The model under review builds one solid part; all positions refer to its coordinate system, in mm. Face numbers are marked on the shaded views. A direction names the side the tool comes from. Round coordinates to 2 decimals unless told otherwise and drop trailing zeros. Write each loop counter-clockwise with the first axis right and the second up, starting at its lowest first coordinate (ties: lowest second). Pieces come first, ordered by that corner, then holes. Notation, with made-up numbers: (17.25, 14) -> (53.25, 14) arc R23 ccw to (53.25, 31) -> close; hole circle Ø11 at (-9.5, 32.25). An arc over 180 degrees is marked (long way). Answer as a JSON object with one key per item and string values. Group by question number.
1) Machinability: for the marked faces 1, 2, 3 and 4, which of the approach directions +Z, -Z, +X, -X, +Y, -Y give a long, thin tool a straight path to every point of the face, cutting with its end or side? Answer none if there is none.
2) Mouldability with a two-part tool opening along X and no side actions: class the marked faces 5, 6 and 7 as pulls with the +X half, pulls with the -X half, needs draft (parallel to the pull), parting line crosses it, or undercut.
3) We need section D-D, the plane y = -4.25. Write out the cut boundary in (x, z), then the cut area to 3 significant figures.
4) We need section C-C, the plane z = 0.5. Write out the cut boundary in (x, y), then the cut area to 3 significant figures.
5) We need section B-B, the plane x = 0. Write out the cut boundary in (y, z), then the cut area to 3 significant figures.
6) Insertion check: pin 1 Ø1.5 at (y, z) = (-5, -2) entering from -X; pin 2 Ø5.5 at (y, z) = (4, -1) entering from +X; pin 3 Ø1.5 at (y, z) = (-5.5, -2) entering from +X; pin 4 Ø1.2 at (x, y) = (-11, 0) entering from -Z. Each pin has a flat end and moves straight along its axis. Give the tip position at first contact, or say it passes through.
7) To check wall thickness, follow probe 1 along Y at (x, z) = (3, -4); probe 2 along Y at (x, z) = (-11, -1.55); probe 3 along Z at (x, y) = (7.5, 6.25). State the ranges of each line that lie inside material, in increasing order. Write a range as [from, to].
8) We need section A-A, the plane y = 0. Write out the cut boundary in (x, z), then the cut area to 3 significant figures.
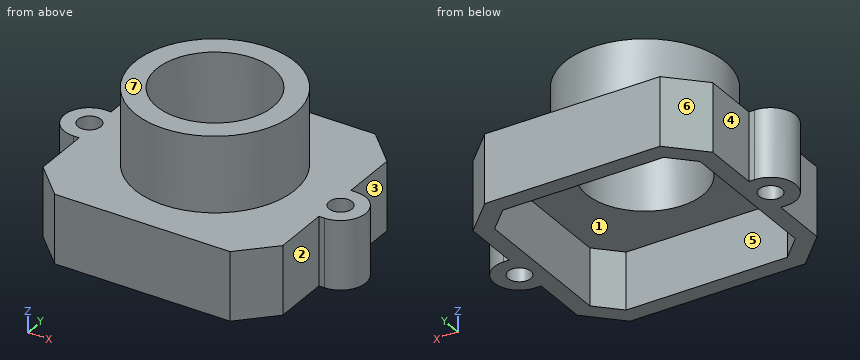
from build123d import *

# Parameters (mm, degrees)
SKETCH1_R                = 1
ROOF_DEPTH               = 1
WALLS_START              = -5
SKETCH1_3_R              = 1
WALLS_DEPTH              = 5
SKETCH2_R                = 5.1
SCREW_HOLE_IN_ROOF_DEPTH = 18.613631253
SCREW_START              = 6.6
SKETCH2_3_R              = 7
SKETCH2_3_R_2            = 5.1
SCREW_HOLDER_DEPTH       = 6.6


with BuildPart() as part:
    # Sketch1 → Roof (new body)
    with BuildSketch(Plane.XY):
        with BuildLine():
            Line((-7.67766953, 10), (-10.5, 7.17766953))
            Line((-10.5, 7.17766953), (-10.5, 2.2))
            Line((-10.5, 2.2), (-11.000000224, 2.2))
            ThreePointArc((-11.000000224, 2.2), (-13.200000224, 0), (-11.000000224, -2.2))
            Line((-11.000000224, -2.2), (-10.5, -2.2))
            Line((-10.5, -2.2), (-10.5, -7.17766953))
            Line((-10.5, -7.17766953), (-7.67766953, -10))
            Line((-7.67766953, -10), (7.67766953, -10))
            Line((7.67766953, -10), (10.5, -7.17766953))
            Line((10.5, -7.17766953), (10.5, -2.2))
            Line((10.5, -2.2), (11, -2.2))
            ThreePointArc((11, -2.2), (13.2, 0), (11, 2.2))
            Line((11, 2.2), (10.5, 2.2))
            Line((10.5, 2.2), (10.5, 7.17766953))
            Line((10.5, 7.17766953), (7.67766953, 10))
            Line((7.67766953, 10), (-7.67766953, 10))
        make_face()
        with Locations((11, 0)):
            Circle(SKETCH1_R, mode=Mode.SUBTRACT)
        with Locations((-11.000000224, 0)):
            Circle(SKETCH1_R, mode=Mode.SUBTRACT)
    extrude(amount=ROOF_DEPTH)

    # Sketch1<3> → Walls (add)
    with BuildSketch(Plane.XY.offset(WALLS_START)):
        with BuildLine():
            Line((-7.67766953, 10), (-10.5, 7.17766953))
            Line((-10.5, 7.17766953), (-10.5, 2.2))
            Line((-10.5, 2.2), (-11.000000224, 2.2))
            ThreePointArc((-11.000000224, 2.2), (-13.200000224, 0), (-11.000000224, -2.2))
            Line((-11.000000224, -2.2), (-10.5, -2.2))
            Line((-10.5, -2.2), (-10.5, -7.17766953))
            Line((-10.5, -7.17766953), (-7.67766953, -10))
            Line((-7.67766953, -10), (7.67766953, -10))
            Line((7.67766953, -10), (10.5, -7.17766953))
            Line((10.5, -7.17766953), (10.5, -2.2))
            Line((10.5, -2.2), (11, -2.2))
            ThreePointArc((11, -2.2), (13.2, 0), (11, 2.2))
            Line((11, 2.2), (10.5, 2.2))
            Line((10.5, 2.2), (10.5, 7.17766953))
            Line((10.5, 7.17766953), (7.67766953, 10))
            Line((7.67766953, 10), (-7.67766953, 10))
        make_face()
        with Locations((11, 0)):
            Circle(SKETCH1_3_R, mode=Mode.SUBTRACT)
        with Locations((-11.000000224, 0)):
            Circle(SKETCH1_3_R, mode=Mode.SUBTRACT)
        Polygon((-9, -6.556349186), (-9, 6.556349186), (-7.056349186, 8.5), (7.056349186, 8.5), (9, 6.556349186), (9, -6.556349186), (7.056349186, -8.5), (-7.056349186, -8.5), align=None, mode=Mode.SUBTRACT)
    extrude(amount=WALLS_DEPTH)

    # Sketch2 → Screw hole in roof (cut, through all)
    with BuildSketch(Plane.XY.offset(1)):
        Circle(SKETCH2_R)
    extrude(amount=-SCREW_HOLE_IN_ROOF_DEPTH, mode=Mode.SUBTRACT)

    # Sketch2<3> → Screw holder (add)
    with BuildSketch(Plane.XY.offset(1).offset(SCREW_START)):
        Circle(SKETCH2_3_R)
        Circle(SKETCH2_3_R_2, mode=Mode.SUBTRACT)
    extrude(amount=-SCREW_HOLDER_DEPTH)


solid = part.part
Here are the results:
{
 "1": {"face 1": "-Z", "face 2": "+Z, -Z, +X, -Y", "face 3": "+Z, -Z, +X, +Y", "face 4": "+Z, -Z, -X, +Y"},
 "2": {"face 5": "undercut", "face 6": "pulls with the -X half", "face 7": "needs draft"},
 "3": {"outline": "(-10.5, -5) -> (-9, -5) -> (-9, 0) -> (-2.82, 0) -> (-2.82, 7.6) -> (-5.56, 7.6) -> (-5.56, 1) -> (-10.5, 1) -> close; (2.82, 0) -> (9, 0) -> (9, -5) -> (10.5, -5) -> (10.5, 1) -> (5.56, 1) -> (5.56, 7.6) -> (2.82, 7.6) -> close", "area": "66.6 mm^2"},
 "4": {"outline": "(-11, -2.2) -> (-10.5, -2.2) -> (-10.5, -7.18) -> (-7.68, -10) -> (7.68, -10) -> (10.5, -7.18) -> (10.5, -2.2) -> (11, -2.2) arc R2.2 ccw to (11, 2.2) -> (10.5, 2.2) -> (10.5, 7.18) -> (7.68, 10) -> (-7.68, 10) -> (-10.5, 7.18) -> (-10.5, 2.2) -> (-11, 2.2) arc R2.2 ccw to start; hole circle Ø2 at (-11, 0); hole circle Ø10.2 at (0, 0); hole circle Ø2 at (11, 0)", "area": "336 mm^2"},
 "5": {"outline": "(-10, -5) -> (-8.5, -5) -> (-8.5, 0) -> (-5.1, 0) -> (-5.1, 7.6) -> (-7, 7.6) -> (-7, 1) -> (-10, 1) -> close; (5.1, 0) -> (8.5, 0) -> (8.5, -5) -> (10, -5) -> (10, 1) -> (7, 1) -> (7, 7.6) -> (5.1, 7.6) -> close", "area": "49.9 mm^2"},
 "6": {"pin 1": "stops at x = -10.5", "pin 2": "stops at x = 12.81", "pin 3": "stops at x = 10.5", "pin 4": "passes through"},
 "7": {"probe 1": "y = [-10, -8.5], [8.5, 10]", "probe 2": "y = [-2.2, -1], [1, 2.2]", "probe 3": "z = [0, 1]"},
 "8": {"outline": "(-13.2, -5) -> (-12, -5) -> (-12, 1) -> (-13.2, 1) -> close; (-10, -5) -> (-9, -5) -> (-9, 0) -> (-5.1, 0) -> (-5.1, 7.6) -> (-7, 7.6) -> (-7, 1) -> (-10, 1) -> close; (5.1, 0) -> (9, 0) -> (9, -5) -> (10, -5) -> (10, 1) -> (7, 1) -> (7, 7.6) -> (5.1, 7.6) -> close; (12, -5) -> (13.2, -5) -> (13.2, 1) -> (12, 1) -> close", "area": "59.3 mm^2"}
}
